Build history of the part. All positions in model axes, mm. A direction names the side the tool comes from. Coordinates: 2 decimals unless noted, no trailing zeros. Loops run counter-clockwise (first coordinate to the right, second up) from the corner with the lowest first, then second, coordinate; pieces in that order, holes last.
(1) Tool access for faces 4 (the face through (0, 3, 0)), 5 (the face through (-11, 0, 0)): list every direction of +Z, -Z, +X, -X, +Y, -Y with a clear straight run to the whole face (end or side of a thin tool).
(2) Slice it at C-C (x = -7.5). Give the cut face in (y, z), and give its area (3 significant figures).
(3) Wall check: L1, parallel to X at y = 2.25, z = 3; L2, parallel to X at y = 2, z = 4.25; L3, parallel to Y at x = -5.25, z = 0. Give the ranges that are in metal, low to high.
(4) Flat gauge pins, fed straight in: P1, Ø5, axis at x = 7, y = -3.5, coming from the +Z side; P2, Ø4, axis at x = -2.5, z = 2, coming from the -Y side; P3, Ø6, axis at x = 2, y = -0.5, coming from the -Z side. Where does each tip first touch, or does it go through?
(5) Two-plate mould, pull along X, no slides. Class faces 1 (the face through (-9.01, 1.08, 4.88)), 2 (the face through (8, -3.3, -0.1)), 3 (the face through (11, 0, 0)): pulls with the +X half, pulls with the -X half, needs draft (parallel to the pull), parting line crosses it, or undercut.
(6) Slice it at A-A (y = 0). Give the cut face in (x, z), and give its area (3 significant figures).
from build123d import *


with BuildPart() as part:
    # Esquisse1 → Révolution1 (revolve)
    with BuildSketch(Plane.XY):
        Polygon((-11, 0), (11, 0), (11, -4), (10, -5), (8, -5), (8, -3), (-8, -3), (-8, -5), (-10, -5), (-11, -4), align=None)
    revolve(axis=Axis((-11, 0, 0), (1, 0, 0)))


solid = part.part
Response values:
1. face 4: none
1. face 5: +Z, -Z, -X, +Y, -Y
2. outline: circle Ø6 at (0, 0)
2. area: 28.3 mm2
3. L1: x = -11 to -8, 8 to 11
3. L2: x = -10.3 to -8, 8 to 10.3
3. L3: y = -3 to 3
4. P1: stops at z = 4.85
4. P2: stops at y = -3
4. P3: stops at z = -3
5. face 1: needs draft
5. face 2: undercut
5. face 3: pulls with the +X half
6. outline: (-11, -4) - (-10, -5) - (-8, -5) - (-8, -3) - (8, -3) - (8, -5) - (10, -5) - (11, -4) - (11, 4) - (10, 5) - (8, 5) - (8, 3) - (-8, 3) - (-8, 5) - (-10, 5) - (-11, 4) - close
6. area: 154 mm2
